Could you check a few things on this model? Use its own coordinates, in mm. Face numbers are marked on the shaded views. A direction names the side the tool comes from. Coordinates: 2 decimals unless noted, no trailing zeros. Order: outer loops, then holes, each group sorted by start corner. A loop starts at its lowest first (then second) coordinate and runs counter-clockwise, first axis right, second up. Notation, with made-up numbers: (39, -30.75) -> (87, -30.75) arc R11 cw to (87, -9.75) -> close; hole circle Ø7 at (72, 68). An arc over 180 degrees is marked (long way). Put each result on its own line as item: value. Start each with the question number.
Q1. For the marked faces 3 and 4, which set-ups out of +Z, -Z, +X, -X, +Y, -Y let a thin tool reach every point of the face, with its end or its side?
Q2. If we section it at B-B (z = -43): Please give me the cut outline in (x, y), and give its area (3 significant figures).
Q3. If we section it at D-D (x = 31): Please give me the cut outline in (y, z), and give its area (3 significant figures).
Q4. If we section it at C-C (y = -57): Please give me the cut outline in (x, z).
Q5. Please list where these lines run through material, in increasing order: line 1 along Y through (x, z) = (28, 2); line 2 along Z through (x, y) = (0, -65); line 3 along Z through (x, y) = (17, -14).
Q6. If we section it at A-A (x = 0): Please give me the cut outline in (y, z).
Q7. Will these pins go through, and if not, where does the flat tip stop? pin 1 (8 mm diameter, centred on x = -39.5, y = -28, fed in from -Z); pin 2 (5.5 mm diameter, centred on y = -66, z = 43.5, fed in from -X); pin 3 (1 mm diameter, centred on x = 14.5, y = -39.5, fed in from -Z); pin 4 (1.5 mm diameter, centred on y = -65.5, z = 45.5, fed in from +X).
Q8. We'd pull the mould along X, two halves only. Please class the marked faces 1 and 2: +X half, -X half, draft (parallel to the pull), parting line (faces both ways), or undercut.
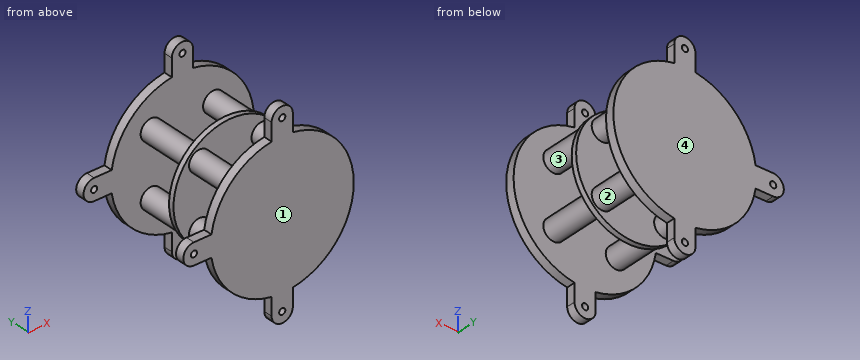
Autodesk Inventor part; units mm, degrees
ref_plane "YZ Plane" through (0, 0, 0) normal (1, 0, 0) x (0, 1, 0)
ref_plane "XZ Plane" through (0, 0, 0) normal (0, 1, 0) x (-1, 0, 0)
ref_plane "XY Plane" through (0, 0, 0) normal (0, 0, 1) x (1, 0, 0)
sketch "Sketch1" plane through (0, 0, 0) normal (0, 1, 0) x (-1, 0, 0)
  circle A0 centre (0, 0) radius 40.5
  circle A1 centre (0, 0) radius 39
  line L0 (0, 50) -> (0, -50) construction
  arc A2 (6, 50) -> (-6, 50) centre (0, 50) ccw
  arc A3 (-6, -50) -> (6, -50) centre (0, -50) ccw
  line L1 (0, 0) -> (50, 0) construction
  arc A4 (50, -6) -> (50, 6) centre (50, 0) ccw
  line L2 (0, 0) -> (50, 0) construction
  line L3 (50, 6) -> (40.0531, 6)
  line L4 (40.0531, -6) -> (50, -6)
  line L5 (6, 40.0531) -> (6, 50)
  line L6 (-6, 50) -> (-6, 40.0531)
  line L7 (-6, -40.0531) -> (-6, -50)
  line L8 (6, -50) -> (6, -40.0531)
  circle A5 centre (50, 0) radius 1.75
  circle A6 centre (0, -50) radius 1.75
  circle A7 centre (0, 50) radius 1.75
  point P0 (25, 0)
  dimension "d0" = 81
  dimension "d1" = 78
  dimension "d2" = 100
  dimension "d3" = 12
  dimension "d4" = 50
  dimension "d5" = 50
  dimension "d6" = 0
  dimension "d7" = 12
  dimension "d8" = 3.5
  dimension "d9" = 3.5
  dimension "d10" = 3.5
extrude "Extrusion1" add sketch "Sketch1" along normal blind 5 contours A0 | A0 L3 A4 L4 | A0 L6 A2 L5 | L8 A3 L7 A0 | A1
sketch "Sketch2" plane through (0, 0, 0) normal (0, -1, 0) x (1, 0, 0)
  line L0 (0, 0) -> (-17.6777, -17.6777)
  line L1 (0, 0) -> (25, 0) construction
  circle A0 centre (-17.6777, -17.6777) radius 6
  circle A1 centre (17.6777, -17.6777) radius 6
  circle A2 centre (17.6777, 17.6777) radius 6
  circle A3 centre (-17.6777, 17.6777) radius 6
  circle A4 centre (17.6777, -17.6777) radius 2
  circle A5 centre (-17.6777, -17.6777) radius 2
  circle A6 centre (17.6777, 17.6777) radius 2
  circle A7 centre (-17.6777, 17.6777) radius 2
  dimension "d13" = 25
  dimension "d14" = 135
  dimension "d15" = 12
  dimension "d18" = 360
  dimension "d22" = 4
  dimension "d23" = 4
  dimension "d24" = 4
  dimension "d25" = 4
extrude "Extrusion2" add sketch "Sketch2" along normal blind 30
sketch "Sketch3" plane through (-17.6777, -30, 17.6777) normal (0, -1, 0) x (1, 0, 0)
  circle A0 centre (17.6777, -17.6777) radius 32.5
  dimension "d26" = 65
extrude "Extrusion3" add sketch "Sketch3" along normal blind 3
sketch "Sketch4" plane through (0, -33, 0) normal (0, -1, 0) x (1, 0, 0)
  circle A0 centre (17.6777, 17.6777) radius 6
  circle A1 centre (17.6777, 17.6777) radius 2
  circle A2 centre (17.6777, -17.6777) radius 2
  circle A3 centre (17.6777, -17.6777) radius 6
  circle A4 centre (-17.6777, 17.6777) radius 2
  circle A5 centre (-17.6777, 17.6777) radius 6
  circle A6 centre (-17.6777, -17.6777) radius 2
  circle A7 centre (-17.6777, -17.6777) radius 6
  point P0 (0, 0)
extrude "Extrusion4" add sketch "Sketch4" along normal blind 30
sketch "Sketch5" plane through (17.6777, -63, -17.6777) normal (0, -1, 0) x (1, 0, 0)
  circle A0 centre (0, 35.3553) radius 6
  circle A1 centre (-35.3553, 0) radius 6
  circle A2 centre (0, 0) radius 6
  circle A3 centre (-35.3553, 35.3553) radius 6
  circle A4 centre (-67.6777, 17.6777) radius 1.75
  circle A5 centre (-17.6777, -32.3223) radius 1.75
  circle A6 centre (-17.6777, 67.6777) radius 1.75
  arc A7 (-23.6777, -32.3223) -> (-11.6777, -32.3223) centre (-17.6777, -32.3223) ccw
  line L0 (-11.6777, -22.3754) -> (-11.6777, -32.3223)
  arc A8 (-11.6777, -22.3754) -> (-11.6777, 57.7308) centre (-17.6777, 17.6777) ccw
  line L1 (-11.6777, 67.6777) -> (-11.6777, 57.7308)
  arc A9 (-11.6777, 67.6777) -> (-23.6777, 67.6777) centre (-17.6777, 67.6777) ccw
  line L2 (-23.6777, 57.7308) -> (-23.6777, 67.6777)
  arc A10 (-23.6777, 57.7308) -> (-57.7308, 23.6777) centre (-17.6777, 17.6777) ccw
  line L3 (-67.6777, 23.6777) -> (-57.7308, 23.6777)
  arc A11 (-67.6777, 23.6777) -> (-67.6777, 11.6777) centre (-67.6777, 17.6777) ccw
  line L4 (-57.7308, 11.6777) -> (-67.6777, 11.6777)
  arc A12 (-57.7308, 11.6777) -> (-23.6777, -22.3754) centre (-17.6777, 17.6777) ccw
  line L5 (-23.6777, -32.3223) -> (-23.6777, -22.3754)
extrude "Extrusion5" add sketch "Sketch5" along normal blind 5 contours A0 | A1 | A2 | A3 | L5 A12 L4 A11 L3 A10 L2 A9 L1 A8 L0 A7
properties part number "Height_upgrade"
The answers:
1. face 3: none
1. face 4: +Z, -Z, +X, -X, +Y
2. outline: (-6, -68) -> (6, -68) -> (6, -63) -> (-6, -63) -> close; (-6, 0) -> (6, 0) -> (6, 5) -> (-6, 5) -> close
2. area: 120 mm^2
3. outline: (-68, -26.06) -> (-63, -26.06) -> (-63, 26.06) -> (-68, 26.06) -> close; (-33, -9.76) -> (-30, -9.76) -> (-30, 9.76) -> (-33, 9.76) -> close; (0, -26.06) -> (5, -26.06) -> (5, 26.06) -> (0, 26.06) -> close
3. area: 580 mm^2
4. outline: circle Ø12 at (-17.68, -17.68); circle Ø12 at (-17.68, 17.68); circle Ø12 at (17.68, -17.68); circle Ø12 at (17.68, 17.68); hole circle Ø4 at (-17.68, -17.68); hole circle Ø4 at (-17.68, 17.68); hole circle Ø4 at (17.68, -17.68); hole circle Ø4 at (17.68, 17.68)
5. line 1: -68 to -63, -33 to -30, 0 to 5
5. line 2: -56 to -51.75, -48.25 to 48.25, 51.75 to 56
5. line 3: -23.64 to -19.56, -15.8 to -11.72, 11.72 to 15.8, 19.56 to 23.64
6. outline: (-68, -56) -> (-63, -56) -> (-63, -51.75) -> (-68, -51.75) -> close; (-68, -48.25) -> (-63, -48.25) -> (-63, 48.25) -> (-68, 48.25) -> close; (-68, 51.75) -> (-63, 51.75) -> (-63, 56) -> (-68, 56) -> close; (-33, -32.5) -> (-30, -32.5) -> (-30, 32.5) -> (-33, 32.5) -> close; (0, -56) -> (5, -56) -> (5, -51.75) -> (0, -51.75) -> close; (0, -48.25) -> (5, -48.25) -> (5, 48.25) -> (0, 48.25) -> close; (0, 51.75) -> (5, 51.75) -> (5, 56) -> (0, 56) -> close
7. pin 1: through
7. pin 2: x = -6
7. pin 3: z = -23.05
7. pin 4: x = 6
8. face 1: draft
8. face 2: undercut
